Autodesk Inventor part; units mm, degrees
ref_plane "YZ Plane" through (0, 0, 0) normal (1, 0, 0) x (0, 1, 0)
ref_plane "XZ Plane" through (0, 0, 0) normal (0, 1, 0) x (-1, 0, 0)
ref_plane "XY Plane" through (0, 0, 0) normal (0, 0, 1) x (1, 0, 0)
sketch "Sketch1" plane through (0, 0, 0) normal (0, 0, 1) x (1, 0, 0)
  circle A0 centre (0, 0) radius 34.75
  dimension "d0" = 69.5
extrude "Extrusion1" add sketch "Sketch1" along normal blind 35
sketch "Sketch2" plane through (0, 0, 35) normal (0, 0, 1) x (1, 0, 0)
  circle A0 centre (0, 0) radius 27.5
  dimension "d3" = 55
extrude "Extrusion2" add sketch "Sketch2" along normal blind 2.5
sketch "Sketch3" plane through (0, 0, 37.5) normal (0, 0, 1) x (1, 0, 0)
  circle A0 centre (0, 0) radius 17
  dimension "d6" = 34
extrude "Extrusion3" cut sketch "Sketch3" against normal blind 18
sketch "Sketch4" plane through (0, 0, 19.5) normal (0, 0, 1) x (1, 0, 0)
  circle A0 centre (0, 0) radius 9.85
  dimension "d9" = 19.7
extrude "Extrusion4" cut sketch "Sketch4" against normal through all
sketch "Sketch5" plane through (0, 0, 0) normal (0, 0, -1) x (-1, 0, 0)
  circle A0 centre (0, 1.85) radius 15
  circle A1 centre (0, 0) radius 9.85
  circle A2 centre (0, 0) radius 34.75
  point P0 (0, -13.15)
  point P1 (0, -9.85)
  point P2 (0, 16.85)
  point P3 (0, 34.75)
  point P4 (0, 9.85)
  dimension "d12" = 30
  dimension "d13" = 3.3
  dimension "d14" = 7
extrude "Extrusion5" add sketch "Sketch5" along normal blind 10 contours A0
sketch "Sketch6" plane through (0, 0, 0) normal (0, 0, -1) x (-1, 0, 0)
  circle A0 centre (0, 0) radius 34.75
  line L0 (0, 34.75) -> (0, -17.55)
  line L1 (-32.813, -17.55) -> (43.7984, -17.55)
  line L2 (43.7984, -17.55) -> (43.7984, -45.8999)
  line L3 (43.7984, -45.8999) -> (-32.813, -45.8999)
  line L4 (-32.813, -45.8999) -> (-32.813, -17.55)
  dimension "d17" = 52.3
extrude "Extrusion6" cut sketch "Sketch6" against normal through all contours L1 L2 L3 L4 A0 | A0 L1
sketch "Sketch7" plane through (0, 0, 37.5) normal (0, 0, 1) x (1, 0, 0)
  circle A0 centre (-6.9364, 19.8214) radius 2.25
  circle A1 centre (19.8214, 6.9364) radius 2.25
  circle A2 centre (-19.8214, -6.9364) radius 2.25
  point P0 (0, 0)
hole "Hole1" at (-6.9364, 19.8214, 37.5) at (-19.8214, -6.9364, 37.5) at (19.8214, 6.9364, 37.5) direction (0, 0, -1) diameter 4.134 depth 14.2 tip angle 118
properties part number "Ross Made spacer"
Here's how the part is built. I have some questions about the finished solid (model axes, mm). A direction names the side the tool comes from. Give positions to 0.01 mm unless a question says otherwise; leave off trailing zeros. Loops run counter-clockwise (first coordinate to the right, second up) from the corner with the lowest first, then second, coordinate; pieces in that order, holes last. Notation, with made-up numbers: (12, -21.75) -> (17, -21.75) arc R14 ccw to (17, 0.25) -> close; hole circle Ø9 at (8, -27.5). An arc over 180 degrees is marked (long way). One line per item, written item: value.
Q1. Suppose I cut it at B-B on y = -3. Please give me the cut outline in (x, z).
Answers follow:
outline: (-34.62, 0) -> (-14.19, 0) -> (-14.19, -10) -> (-9.38, -10) -> (-9.38, 19.5) -> (-16.73, 19.5) -> (-16.73, 37.5) -> (-27.34, 37.5) -> (-27.34, 35) -> (-34.62, 35) -> close; (9.38, -10) -> (14.19, -10) -> (14.19, 0) -> (34.62, 0) -> (34.62, 35) -> (27.34, 35) -> (27.34, 37.5) -> (16.73, 37.5) -> (16.73, 19.5) -> (9.38, 19.5) -> close
Q2. Suppose I cut it at D-D on y = 13. Please give me the cut outline in (x, z).
Answers follow:
outline: (-32.23, 0) -> (-10.03, 0) -> (-10.03, -10) -> (10.03, -10) -> (10.03, 0) -> (32.23, 0) -> (32.23, 35) -> (24.23, 35) -> (24.23, 37.5) -> (10.95, 37.5) -> (10.95, 19.5) -> (-10.95, 19.5) -> (-10.95, 37.5) -> (-24.23, 37.5) -> (-24.23, 35) -> (-32.23, 35) -> close
Q3. We'd pull the mould along X, two halves only. Please class faces 4 (the face through (0.65, 9.83, 4.96)), 5 (the face through (-6, 9, -10)), 6 (the face through (-1.022, 34.735, 17.255)): pulls with the +X half, pulls with the -X half, needs draft (parallel to the pull), parting line crosses it, or undercut.
Answers follow:
face 4: undercut
face 5: needs draft
face 6: parting line crosses it
Q4. Suppose I cut it at C-C on z = -6. Please give me the cut outline in (x, y), then the cut area to 3 significant figures.
Answers follow:
outline: circle Ø30 at (0, 1.85); hole circle Ø19.7 at (0, 0)
area: 402 mm^2
Q5. On a 3-axis mill with a long thin cutter (end or side, diameter ignored), from which of +Z, -Z, +X, -X, +Y, -Y can I reach the whole of each face in a straight line? I mean faces 1 (the face through (14.985, 1.19, -4.93)), 2 (the face through (0, 20, 37.5)), 3 (the face through (9.139, 14.334, 28.626)). Say none if no direction works.
Answers follow:
face 1: -Z
face 2: +Z, +X, -X, +Y, -Y
face 3: +Z
Q6. If I drill on line 1 along Y through (x, z) = (0, 9.75); line 2 along Y through (x, z) = (-27, 30); line 3 along Y through (x, z) = (14, 35.5), over which ranges is the centre line in solid material (lowest first)?
Answers follow:
line 1: -17.55 to -9.85, 9.85 to 34.75
line 2: -17.55 to 21.88
line 3: -17.55 to -9.64, 9.64 to 23.67
Q7. Suppose I cut it at A-A on x = 0. Please give me the cut outline in (y, z).
Answers follow:
outline: (-17.55, 0) -> (-13.15, 0) -> (-13.15, -10) -> (-9.85, -10) -> (-9.85, 19.5) -> (-17, 19.5) -> (-17, 37.5) -> (-17.55, 37.5) -> close; (9.85, -10) -> (16.85, -10) -> (16.85, 0) -> (34.75, 0) -> (34.75, 35) -> (27.5, 35) -> (27.5, 37.5) -> (17, 37.5) -> (17, 19.5) -> (9.85, 19.5) -> close
Q8. I'm going to push flat-ended pins straight in: pin 1 Ø1 at (y, z) = (-8.5, 29.5) entering from -X; pin 2 Ø3.5 at (x, y) = (-19.82, -6.94) entering from +Z; pin 3 Ø2 at (y, z) = (4, 30.5) entering from +X. Where does each tip first touch, or does it pass through?
Answers follow:
pin 1: x = -33.82
pin 2: z = 23.11
pin 3: x = 34.62
